from build123d import *

# Parameters (mm, degrees)
SKETCH1_W           = 62
SKETCH1_H           = 42
SKETCH1_W_2         = 41
SKETCH1_H_2         = 21
BOSS_EXTRUDE1_DEPTH = 43
SKETCH2_W           = 4
SKETCH2_H           = 25
BOSS_EXTRUDE2_DEPTH = 5.5
SKETCH_1_R          = 5
CUT_EXTRUDE_1_DEPTH = 42
SKETCH_2_W          = 41
SKETCH_2_H          = 21
SKETCH_2_R          = 7
EXTRUDE_1_DEPTH     = 1
SKETCH_2_3_W        = 62
SKETCH_2_3_H        = 42
SKETCH_2_3_R        = 7
EXTRUDE_2_DEPTH     = 1
FILLET_1_R          = 4
FILLET_2_R          = 4
FILLET_3_R          = 4
FILLET_4_R          = 4
SKETCH2_3_W         = 4
SKETCH2_3_H         = 25
EXTRUDE_3_DEPTH     = 49.5
EXTRUDE_4_DEPTH     = 0.75
EXTRUDE_5_DEPTH     = 0.75


with BuildPart() as part:
    # Sketch1 → Boss-Extrude1 (new body)
    with BuildSketch(Plane.XY):
        with Locations((1.904162196, -4.136072895)):
            Rectangle(SKETCH1_W, SKETCH1_H)
        with Locations((1.904162196, -4.136072895)):
            Rectangle(SKETCH1_W_2, SKETCH1_H_2, mode=Mode.SUBTRACT)
    extrude(amount=BOSS_EXTRUDE1_DEPTH)

    # Sketch2 → Boss-Extrude2 (add)
    with BuildSketch(Plane.XY.offset(43)):
        with Locations((-27.095837804, -4.136072895)):
            Rectangle(SKETCH2_W, SKETCH2_H)
    extrude(amount=BOSS_EXTRUDE2_DEPTH)

    # Sketch 1 → Cut-Extrude 1 (cut)
    with BuildSketch(Plane(origin=(0, 16.863927105, 0), x_dir=(1, 0, 0), z_dir=(0, 1, 0))):
        with Locations((7.653776732, -32.500385465)):
            Circle(SKETCH_1_R)
    extrude(amount=-CUT_EXTRUDE_1_DEPTH, mode=Mode.SUBTRACT)

    # Sketch 2 → Extrude 1 (add)
    with BuildSketch(Plane(origin=(0, 0, 0), x_dir=(-1, 0, 0), z_dir=(0, 0, -1))):
        with Locations((-1.904162196, -4.136072895)):
            Rectangle(SKETCH_2_W, SKETCH_2_H)
        with Locations((-12.404162196, -4.136072895)):
            Circle(SKETCH_2_R, mode=Mode.SUBTRACT)
    extrude(amount=-EXTRUDE_1_DEPTH)

    # Sketch 2_3 → Extrude 2 (add)
    with BuildSketch(Plane(origin=(0, 0, 0), x_dir=(-1, 0, 0), z_dir=(0, 0, -1))):
        with Locations((-1.904162196, -4.136072895)):
            Rectangle(SKETCH_2_3_W, SKETCH_2_3_H)
        with Locations((-12.404162196, -4.136072895)):
            Circle(SKETCH_2_3_R, mode=Mode.SUBTRACT)
    extrude(amount=EXTRUDE_2_DEPTH)

    # Fillet 1
    fillet_1_edges = [part.edges().sort_by_distance(p)[0] for p in [
        (32.904162196, -25.136072895, 21),
    ]]
    fillet(fillet_1_edges, radius=FILLET_1_R)

    # Fillet 2
    fillet_2_edges = [part.edges().sort_by_distance(p)[0] for p in [
        (-29.095837804, -25.136072895, 21),
    ]]
    fillet(fillet_2_edges, radius=FILLET_2_R)

    # Fillet 3
    fillet_3_edges = [part.edges().sort_by_distance(p)[0] for p in [
        (32.904162196, 16.863927105, 21),
    ]]
    fillet(fillet_3_edges, radius=FILLET_3_R)

    # Fillet 4
    fillet_4_edges = [part.edges().sort_by_distance(p)[0] for p in [
        (-29.095837804, 16.863927105, 21),
    ]]
    fillet(fillet_4_edges, radius=FILLET_4_R)

    # Sketch2_3 → Extrude 3 (add)
    with BuildSketch(Plane.XY.offset(43)):
        with Locations((-27.095837804, -4.136072895)):
            Rectangle(SKETCH2_3_W, SKETCH2_3_H)
    extrude(amount=-EXTRUDE_3_DEPTH)

    # Sketch 5 → Extrude 4 (add)
    with BuildSketch(Plane(origin=(0, -4.136072895, 0), x_dir=(1, 0, 0), z_dir=(0, 1, 0))):
        with BuildLine():
            Line((-29.095837804, -21), (-29.095837804, 6.5))
            ThreePointArc((-29.095837804, 6.5), (-81.244156023, 0.562066252), (-129.095837804, -21))
            Line((-129.095837804, -21), (-29.095837804, -21))
        make_face()
        with BuildLine():
            Line((-29.095837804, -48.5), (-29.095837804, -21))
            Line((-29.095837804, -21), (-129.095837804, -21))
            ThreePointArc((-129.095837804, -21), (-81.244156023, -42.562066252), (-29.095837804, -48.5))
        make_face()
    extrude(amount=EXTRUDE_4_DEPTH)

    # Sketch 5_3 → Extrude 5 (add)
    with BuildSketch(Plane(origin=(0, -4.136072895, 0), x_dir=(1, 0, 0), z_dir=(0, 1, 0))):
        with BuildLine():
            Line((-29.095837804, -21), (-29.095837804, 6.5))
            ThreePointArc((-29.095837804, 6.5), (-81.244156023, 0.562066252), (-129.095837804, -21))
            Line((-129.095837804, -21), (-29.095837804, -21))
        make_face()
        with BuildLine():
            Line((-29.095837804, -48.5), (-29.095837804, -21))
            Line((-29.095837804, -21), (-129.095837804, -21))
            ThreePointArc((-129.095837804, -21), (-81.244156023, -42.562066252), (-29.095837804, -48.5))
        make_face()
    extrude(amount=-EXTRUDE_5_DEPTH)


solid = part.part
The model under review builds one solid part; all positions refer to its coordinate system, in mm. A direction names the side the tool comes from. Round coordinates to 2 decimals unless told otherwise and drop trailing zeros. Order: outer loops, then holes, each group sorted by start corner. A loop starts at its lowest first (then second) coordinate and runs counter-clockwise, first axis right, second up. Notation, with made-up numbers: (78, -10.75) -> (115, -10.75) arc R27 cw to (115, 5.25) -> close; hole circle Ø5 at (10.25, 69). An arc over 180 degrees is marked (long way). Write item = value, one per line. Start each with the question number.
Item 1: For line 1 along X through (y, z) = (-8, 4.5); line 2 along Z through (x, y) = (8, 6.5); line 3 along Y through (x, z) = (21, 16), list the stretches that pass through material, from the lowest coordinate up.
Item 2: Consider section A-A on x = -14.5. Write out the cut boundary in (y, z).
Item 3: For faces 4 (the face through (-27, -16.636, 46)), 5 (the face through (2, -14.636, 22)), 6 (the face through (-29.096, 5, 21)), list the 3-axis set-ups (+Z, -Z, +X, -X, +Y, -Y) from which the entire face can be reached by the end or side of a thin tool; tool diameter is ignored.
Item 4: Consider section B-B on z = 7. Write out the cut boundary in (x, y).
Item 5: Consider section D-D on z = 35. Write out the cut boundary in (x, y).
Item 6: Clearance check with flat-ended pins moving along their axes: pin 1 Ø8 at (y, z) = (3, 11.5) entering from -X; pin 2 Ø21 at (x, y) = (-8, 5.5) entering from -Z; pin 3 Ø8 at (x, z) = (7.65, 32.5) entering from -Y; pin 4 Ø4.5 at (x, y) = (-28, -9.5) entering from +Z. State where each tip first meets the part, or that it passes through.
Item 7: Consider section C-C on y = 4.5. Write out the cut boundary in (x, z).
Item 8: Mouldability with a two-part tool opening along X and no side actions: class faces 1 (the face through (2, 6.364, 22)), 2 (the face through (-27.89, -24, 20.69)), 3 (the face through (2, 16.864, 21)) as released by +X, released by -X, zero draft, split by the parting line, or undercut.
Conclusion:
q1.line_1 = -29.1 to -18.6, 22.4 to 32.9
q1.line_2 = -1 to 27.51, 37.49 to 43
q1.line_3 = -25.14 to -14.64, 6.36 to 16.86
q2.outline = (-25.14, -1) -> (16.86, -1) -> (16.86, 43) -> (6.36, 43) -> (6.36, 1) -> (-14.64, 1) -> (-14.64, 43) -> (-25.14, 43) -> close
q3.face_4 = +Z, +X, -X, -Y
q3.face_5 = +Z
q3.face_6 = +Z, -Z, -X, +Y
q4.outline = (-102.9, -4.89) -> (-29.1, -4.89) -> (-29.1, -21.14) arc R4 ccw to (-25.1, -25.14) -> (28.9, -25.14) arc R4 ccw to (32.9, -21.14) -> (32.9, 12.86) arc R4 ccw to (28.9, 16.86) -> (-25.1, 16.86) arc R4 ccw to (-29.1, 12.86) -> (-29.1, -3.39) -> (-102.9, -3.39) -> close; hole (-18.6, -14.64) -> (22.4, -14.64) -> (22.4, 6.36) -> (-18.6, 6.36) -> close
q5.outline = (-102.9, -4.89) -> (-29.1, -4.89) -> (-29.1, -21.14) arc R4 ccw to (-25.1, -25.14) -> (3.32, -25.14) -> (3.32, -14.64) -> (-18.6, -14.64) -> (-18.6, 6.36) -> (3.32, 6.36) -> (3.32, 16.86) -> (-25.1, 16.86) arc R4 ccw to (-29.1, 12.86) -> (-29.1, -3.39) -> (-102.9, -3.39) -> close; (11.98, -25.14) -> (28.9, -25.14) arc R4 ccw to (32.9, -21.14) -> (32.9, 12.86) arc R4 ccw to (28.9, 16.86) -> (11.98, 16.86) -> (11.98, 6.36) -> (22.4, 6.36) -> (22.4, -14.64) -> (11.98, -14.64) -> close
q6.pin_1 = -29.1
q6.pin_2 = -1
q6.pin_3 = through
q6.pin_4 = 48.5
q7.outline = (-29.1, -6.5) -> (-25.1, -6.5) -> (-25.1, -1) -> (32.9, -1) -> (32.9, 43) -> (22.4, 43) -> (22.4, 1) -> (-18.6, 1) -> (-18.6, 43) -> (-25.1, 43) -> (-25.1, 48.5) -> (-29.1, 48.5) -> close
q8.face_1 = undercut
q8.face_2 = released by -X
q8.face_3 = zero draft
